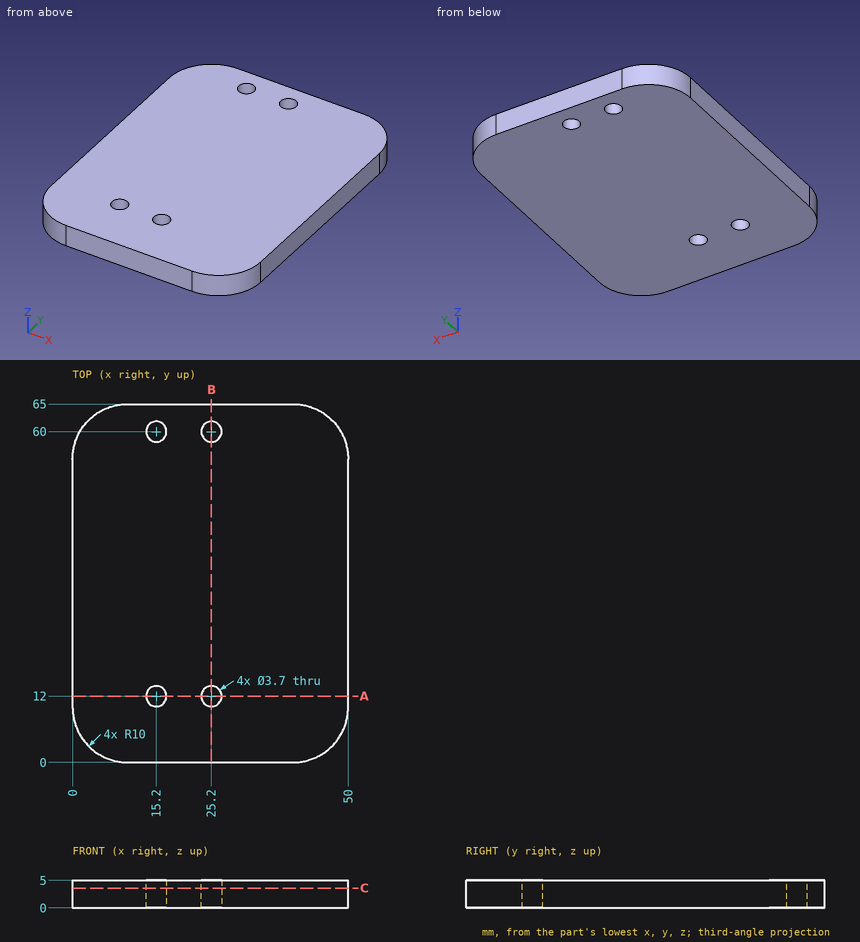
Verification items for this drawing (mm, ordinates from the low corner). Coordinates: 2 decimals unless noted, no trailing zeros. Order: outer loops, then holes, each group sorted by start corner. A loop starts at its lowest first (then second) coordinate and runs counter-clockwise, first axis right, second up. Notation, with made-up numbers: M 74.25,-1 L 120.25,-1 A17 cw 120.25,5 Z; hole C -35,71 d1. An arc over 180 degrees is marked long. One line per item, written item: value. Start each with the question number.
Item 1: Sectioned sample at B-B on x = 25.2. Record the cut outline in (y, z), then the cut area to 3 significant figures.
Item 2: Depth check by flat-ended pin: P1, Ø5, axis at x = 15.2, y = 60, coming from the +Z side. Enter the tip coordinate at first touch or a pass-through.
Item 3: Thickness scan on probe 1 along Y at (x, z) = (25.2, 1.7); probe 2 along X at (y, z) = (61.5, 2.3); probe 3 along Y at (x, z) = (24, 4.3). Record the ranges inside material, lowest first.
Item 4: Sectioned sample at C-C on z = 3.6. Record the cut outline in (x, y).
Item 5: Sectioned sample at A-A on y = 12. Record the cut outline in (x, z), then the cut area to 3 significant figures.
Calculated:
1. outline: M 0,0 L 10.15,0 L 10.15,5 L 0,5 Z; M 13.85,0 L 58.15,0 L 58.15,5 L 13.85,5 Z; M 61.85,0 L 65,0 L 65,5 L 61.85,5 Z
1. area: 288 mm^2
2. P1: z = 5
3. probe 1: 0 to 10.15, 13.85 to 58.15, 61.85 to 65
3. probe 2: 2.4 to 14.12, 16.28 to 24.12, 26.28 to 47.6
3. probe 3: 0 to 10.59, 13.41 to 58.59, 61.41 to 65
4. outline: M 0,10 A10 ccw 10,0 L 40,0 A10 ccw 50,10 L 50,55 A10 ccw 40,65 L 10,65 A10 ccw 0,55 Z; hole C 15.2,12 d3.7; hole C 15.2,60 d3.7; hole C 25.2,12 d3.7; hole C 25.2,60 d3.7
5. outline: M 0,0 L 13.35,0 L 13.35,5 L 0,5 Z; M 17.05,0 L 23.35,0 L 23.35,5 L 17.05,5 Z; M 27.05,0 L 50,0 L 50,5 L 27.05,5 Z
5. area: 213 mm^2
